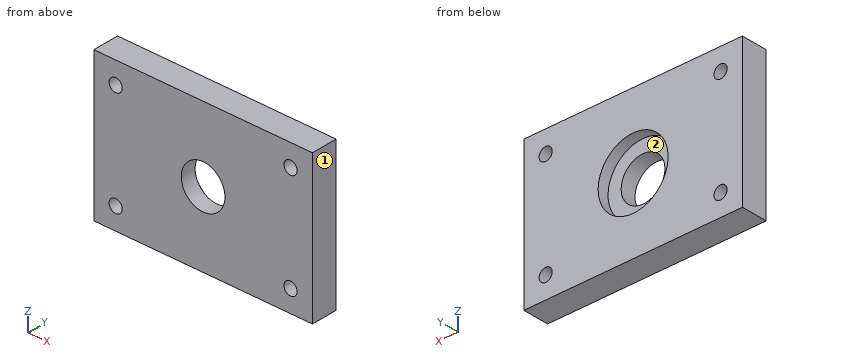
```python
from build123d import *

# Parameters (mm, degrees)
SKETCH1_W                                = 50
SKETCH1_H                                = 34
BEARING_HOLDER_PLATE_BOSS_EXTRUDE1_DEPTH = 6
SKETCH3_R                                = 1.5
MOUNTING_HOLES_CUT_EXTRUDE1_DEPTH        = 6
SKETCH4_R                                = 5
SHAFT_CUT_EXTRUDE2_DEPTH                 = 6
SKETCH5_R                                = 8
BEARING_CUT_EXTRUDE3_DEPTH               = 2.5


with BuildPart() as part:
    # Sketch1 → Bearing Holder Plate Boss-Extrude1 (new body)
    with BuildSketch(Plane(origin=(0, 0, 0), x_dir=(1, 0, 0), z_dir=(0, 1, 0))):
        Rectangle(SKETCH1_W, SKETCH1_H)
    extrude(amount=BEARING_HOLDER_PLATE_BOSS_EXTRUDE1_DEPTH)

    # Sketch3 → Mounting Holes Cut-Extrude1 (cut)
    with BuildSketch(Plane.XZ):
        with Locations(Location((20, 12, 0), (0, 0, 270))):
            Circle(SKETCH3_R)
        with Locations(Location((-20, 12, 0), (0, 0, 270))):
            Circle(SKETCH3_R)
        with Locations(Location((-20, -12, 0), (0, 0, 270))):
            Circle(SKETCH3_R)
        with Locations(Location((20, -12, 0), (0, 0, 270))):
            Circle(SKETCH3_R)
    extrude(amount=-MOUNTING_HOLES_CUT_EXTRUDE1_DEPTH, mode=Mode.SUBTRACT)

    # Sketch4 → Shaft Cut-Extrude2 (cut)
    with BuildSketch(Plane(origin=(0, 6, 0), x_dir=(1, 0, 0), z_dir=(0, 1, 0))):
        with Locations(Location((0, 0, 0), (0, 0, 270))):
            Circle(SKETCH4_R)
    extrude(amount=-SHAFT_CUT_EXTRUDE2_DEPTH, mode=Mode.SUBTRACT)

    # Sketch5 → Bearing Cut-Extrude3 (cut)
    with BuildSketch(Plane(origin=(0, 6, 0), x_dir=(1, 0, 0), z_dir=(0, 1, 0))):
        with Locations(Location((0, 0, 0), (0, 0, 270))):
            Circle(SKETCH5_R)
    extrude(amount=-BEARING_CUT_EXTRUDE3_DEPTH, mode=Mode.SUBTRACT)


solid = part.part
```
Part model, mm, in its own coordinate system. Face numbers are marked on the shaded views. A direction names the side the tool comes from. Give positions to 0.01 mm unless a question says otherwise; leave off trailing zeros. Write each loop counter-clockwise with the first axis right and the second up, starting at its lowest first coordinate (ties: lowest second). Pieces come first, ordered by that corner, then holes. Notation, with made-up numbers: (-21, -6.75) -> (33, -6.75) arc R16 cw to (33, 6.25) -> close; hole circle Ø9 at (10.5, 60.25). An arc over 180 degrees is marked (long way). Put each result on its own line as item: value. Start each with the question number.
Item 1: Cut at B-B (x = -20). List the corners of the cut face in (y, z).
Item 2: Wall check: L1, parallel to X at y = 3.4, z = -12; L2, parallel to X at y = 0.8, z = 0; L3, parallel to X at y = 3.5, z = -11. Give the ranges that are in metal, low to high. Write a range as [from, to].
Item 3: Cut at A-A (z = 12). List the corners of the cut face in (x, y), then the cut area to 3 significant figures.
Item 4: Cut at D-D (z = 0). List the corners of the cut face in (x, y).
Item 5: Cut at C-C (x = 0). List the corners of the cut face in (y, z), then the cut area to 3 significant figures.
Item 6: Which spindle directions (+Z, -Z, +X, -X, +Y, -Y) get a long thin tool onto all of the face, cutting with end or side? Do the marked faces 1 and 2. Say none if no direction does.
Answer list:
1. outline: (0, -17) -> (6, -17) -> (6, -13.5) -> (0, -13.5) -> close; (0, -10.5) -> (6, -10.5) -> (6, 10.5) -> (0, 10.5) -> close; (0, 13.5) -> (6, 13.5) -> (6, 17) -> (0, 17) -> close
2. L1: x = [-25, -21.5], [-18.5, 18.5], [21.5, 25]
2. L2: x = [-25, -5], [5, 25]
2. L3: x = [-25, -21.12], [-18.88, 18.88], [21.12, 25]
3. outline: (-25, 0) -> (-21.5, 0) -> (-21.5, 6) -> (-25, 6) -> close; (-18.5, 0) -> (18.5, 0) -> (18.5, 6) -> (-18.5, 6) -> close; (21.5, 0) -> (25, 0) -> (25, 6) -> (21.5, 6) -> close
3. area: 264 mm2
4. outline: (-25, 0) -> (-5, 0) -> (-5, 3.5) -> (-8, 3.5) -> (-8, 6) -> (-25, 6) -> close; (5, 0) -> (25, 0) -> (25, 6) -> (8, 6) -> (8, 3.5) -> (5, 3.5) -> close
5. outline: (0, -17) -> (6, -17) -> (6, -8) -> (3.5, -8) -> (3.5, -5) -> (0, -5) -> close; (0, 5) -> (3.5, 5) -> (3.5, 8) -> (6, 8) -> (6, 17) -> (0, 17) -> close
5. area: 129 mm2
6. face 1: +Z, -Z, +X, +Y, -Y
6. face 2: +Y
